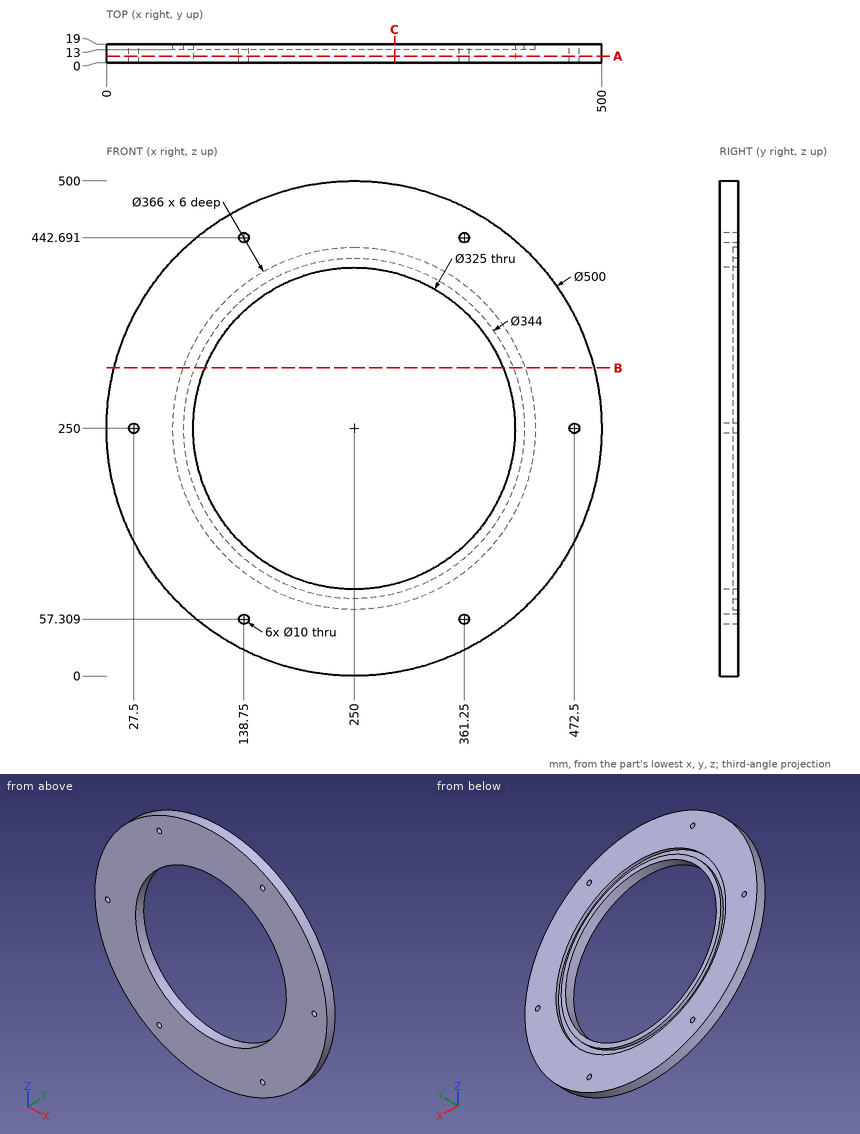
Geometry check sheet. Reference: drawing and pictorial views, mm from the part's lowest x, y, z. Coordinates: 2 decimals unless noted, no trailing zeros. Order: outer loops, then holes, each group sorted by start corner. A loop starts at its lowest first (then second) coordinate and runs counter-clockwise, first axis right, second up.
Item 1: Scan lines: line 1 along X through (y, z) = (10.75, 250); line 2 along X through (y, z) = (16.2, 250); line 3 along Z through (x, y) = (361.25, 8.25) (1 decimal). Record each from-to range of solid material in increasing order.
Item 2: Section check B-B (z = 311). Enter the section's corners in (x, y).
Item 3: Section check A-A (y = 6.75). Enter the section's corners in (x, z).
Item 4: Section check C-C (x = 291). Enter the section's corners in (y, z) (1 decimal).
Item 5: Depth check by flat-ended pin: pin 1 (6 mm diameter, centred on x = 168, y = 4.5, fed in from -Z); pin 2 (10 mm diameter, centred on x = 129.5, y = 8.5, fed in from -Z); pin 3 (1.5 mm diameter, centred on y = 16, z = 137.5, fed in from -X). Enter the tip coordinate at first touch or a pass-through.
Check sheet entries:
1. line 1: x = 0 to 22.5, 32.5 to 87.5, 412.5 to 467.5, 477.5 to 500
1. line 2: x = 0 to 22.5, 32.5 to 67, 78 to 87.5, 412.5 to 422, 433 to 467.5, 477.5 to 500
1. line 3: z = 26.1 to 52.3, 62.3 to 131.6, 368.4 to 437.7, 447.7 to 473.9
2. outline: (7.56, 0) - (99.38, 0) - (99.38, 19) - (89.18, 19) - (89.18, 13) - (77.47, 13) - (77.47, 19) - (7.56, 19) - close; (400.62, 0) - (492.44, 0) - (492.44, 19) - (422.53, 19) - (422.53, 13) - (410.82, 13) - (410.82, 19) - (400.62, 19) - close
3. outline: circle Ø500 at (250, 250); hole circle Ø10 at (27.5, 250); hole circle Ø325 at (250, 250); hole circle Ø10 at (138.75, 57.31); hole circle Ø10 at (138.75, 442.69); hole circle Ø10 at (361.25, 57.31); hole circle Ø10 at (361.25, 442.69); hole circle Ø10 at (472.5, 250)
4. outline: (0, 3.4) - (19, 3.4) - (19, 71.7) - (13, 71.7) - (13, 83) - (19, 83) - (19, 92.8) - (0, 92.8) - close; (0, 407.2) - (19, 407.2) - (19, 417) - (13, 417) - (13, 428.3) - (19, 428.3) - (19, 496.6) - (0, 496.6) - close
5. pin 1: stops at z = 12.81
5. pin 2: stops at z = 28.28
5. pin 3: stops at x = 26.37
